from build123d import *

# Parameters (mm, degrees)
BOSS_EXTRUDE1_DEPTH   = 3
M6_TAPPED_HOLE1_D     = 5
M6_TAPPED_HOLE1_DEPTH = 10
M6_TAPPED_HOLE1_TIP   = 1.502151548


with BuildPart() as part:
    # Sketch1 → Boss-Extrude1 (new body)
    with BuildSketch(Plane(origin=(0, 0, 0), x_dir=(1, 0, 0), z_dir=(0, 1, 0))):
        Polygon((6.92820323, 0), (3.464101615, 6), (-3.464101615, 6), (-6.92820323, 0), (-3.464101615, -6), (3.464101615, -6), align=None)
    extrude(amount=BOSS_EXTRUDE1_DEPTH)

    # Sketch2 → Revolve1 (revolve)
    with BuildSketch(Plane.XY):
        with BuildLine():
            Line((0, 3), (0, 13.5))
            ThreePointArc((0, 13.5), (4.041757337, 8.926634796), (5.5, 3))
            Line((5.5, 3), (0, 3))
        make_face()
    revolve(axis=Axis((0, 3, 0), (0, 1, 0)))

    # M6 Tapped Hole1
    with Locations(Plane(origin=(0, 0, 0), x_dir=(-1, 0, 0), z_dir=(0, -1, 0))):
        with Locations((0, 0)):
            Hole(M6_TAPPED_HOLE1_D / 2, depth=M6_TAPPED_HOLE1_DEPTH)
            with Locations((0, 0, -(M6_TAPPED_HOLE1_DEPTH + M6_TAPPED_HOLE1_TIP / 2))):  # 118° drill point
                Cone(0, M6_TAPPED_HOLE1_D / 2, M6_TAPPED_HOLE1_TIP, mode=Mode.SUBTRACT)


solid = part.part
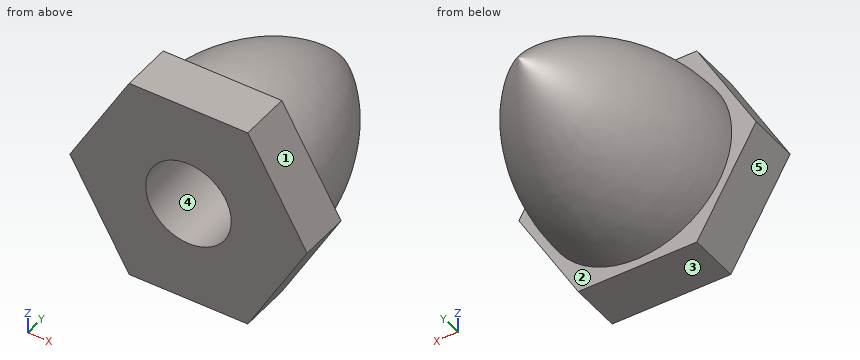
Model file for the job. Use its own axes, mm. Face numbers are marked on the shaded views. A direction names the side the tool comes from. Give positions to 0.01 mm unless a question says otherwise; leave off trailing zeros. Loops run counter-clockwise (first coordinate to the right, second up) from the corner with the lowest first, then second, coordinate; pieces in that order, holes last.
1) Saw through at A-A (y = 1.25). Write the cut outline in (x, z), plus the area to 3 significant figures.
2) Tool access for the marked faces 1 and 2: list every direction of +Z, -Z, +X, -X, +Y, -Y with a clear straight run to the whole face (end or side of a thin tool).
3) Pull direction X, two halves, no side cores. Call the marked faces 3, 4 and 5: +X half, -X half, draft (parallel to the pull), parting line (faces both ways), or undercut.
4) Wall check: line 1 (Z direction, x = 0, y = 2); line 2 (Z direction, x = 0, y = 7); line 3 (X direction, y = 11, z = 0.25). Give the ranges that are in metal, low to high.
5) Flat gauge pins, fed straight in: pin 1 Ø1.5 at (x, y) = (3.5, 9.5) entering from +Z; pin 2 Ø6 at (y, z) = (5.5, -2) entering from +X; pin 3 Ø1.5 at (y, z) = (10.5, -0.5) entering from +X; pin 4 Ø6 at (x, y) = (-5, 4.5) entering from +Z. Where does each tip first touch, or does it go through?
Answer block:
1. outline: (-6.93, 0) - (-3.46, -6) - (3.46, -6) - (6.93, 0) - (3.46, 6) - (-3.46, 6) - close; hole circle Ø5 at (0, 0)
1. area: 105 mm2
2. face 1: +Z, +X, +Y, -Y
2. face 2: +Y
3. face 3: draft
3. face 4: undercut
3. face 5: -X half
4. line 1: z = -6 to -2.5, 2.5 to 6
4. line 2: z = -4.86 to -2.5, 2.5 to 4.86
4. line 3: x = -2.67 to -0.8, 0.8 to 2.67
5. pin 1: stops at z = 2.72
5. pin 2: stops at x = 6.73
5. pin 3: stops at x = 3.54
5. pin 4: stops at z = 6
